```python
from build123d import *

# Parameters (mm, degrees)
F0_W           = 140
F0_H           = 30
F1_DEPTH       = 8
F2_R           = 8.25
F3_DEPTH       = 2
F5_D           = 9
F5_CSINK_D     = 16.5
F5_CSINK_ANGLE = 90
F6_R           = 4
F7_DEPTH       = 55
F8_R           = 2
F10_D          = 6


with BuildPart() as f1:
    # F0 (on Top) → F1 (new body)
    with BuildSketch(Plane.XY):
        Rectangle(F0_W, F0_H)
    extrude(amount=F1_DEPTH)

    # F2 (on face) → F3 (cut)
    with BuildSketch(Plane.XY.offset(8)):
        with Locations((-55, 0)):
            Circle(F2_R)
        Circle(F2_R)
        with Locations((55, 0)):
            Circle(F2_R)
    extrude(amount=-F3_DEPTH, mode=Mode.SUBTRACT)

    # F5 (through all)
    with Locations(Plane.XY.offset(6)):
        with Locations((-55, 0), (0, 0), (55, 0)):
            CounterSinkHole(F5_D / 2, F5_CSINK_D / 2, counter_sink_angle=F5_CSINK_ANGLE)

    # F6 (on Right) → F7 (cut, symmetric)
    with BuildSketch(Plane.YZ):
        with Locations((0, 8)):
            Circle(F6_R)
    extrude(amount=F7_DEPTH, both=True, mode=Mode.SUBTRACT)

    # F8
    f8_edges = [f1.edges().sort_by_distance(p)[0] for p in [
        (-27.5, 4, 8),
        (27.5, 4, 8),
        (27.5, -4, 8),
        (-27.5, -4, 8),
    ]]
    fillet(f8_edges, radius=F8_R)

    # F10 (through all)
    with Locations(Plane.XY.offset(8)):
        with Locations((-40, 0), (40, 0)):
            Hole(F10_D / 2)


solid = f1.part
```
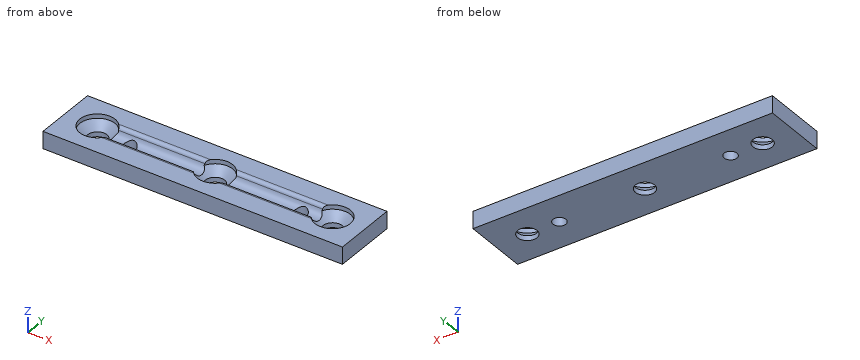
Could you check a few things on this model? Use its own coordinates, in mm. Give positions to 0.01 mm unless a question says otherwise; leave off trailing zeros. Order: outer loops, then holes, each group sorted by start corner. A loop starts at its lowest first (then second) coordinate and runs counter-clockwise, first axis right, second up.
Q1. If I drill on line 1 along X through (y, z) = (0, 0.55); line 2 along Y through (x, z) = (-55, 0.9); line 3 along X through (y, z) = (0, 7.1), over which ranges is the centre line in solid material (lowest first)?
Q2. I'm going to push flat-ended pins straight in: P1, Ø11.5, axis at x = 55, y = 0, coming from the -Z side; P2, Ø7, axis at x = 40, y = 0, coming from the +Z side; P3, Ø5.5, axis at x = -40, y = 0, coming from the +Z side; P4, Ø15, axis at x = 55, y = 0, coming from the +Z side. Where does each tip first touch, or does it pass through?
Q3. Suppose I cut it at B-B, the plane y = 0. Count the separate pieces of the cut face and the enclosed holes in it, and give its area (3 significant figures).
Q4. Suppose I cut it at C-C, the plane x = 40. Write out the boundary of the cut face in (y, z), and give its area (3 significant figures).
Q5. Suppose I cut it at A-A, the plane x = 0. Write out the boundary of the cut face in (y, z), and give its area (3 significant figures).
Solution:
1. line 1: x = -70 to -59.5, -50.5 to -43, -37 to -4.5, 4.5 to 37, 43 to 50.5, 59.5 to 70
1. line 2: y = -15 to -4.5, 4.5 to 15
1. line 3: x = -70 to -63.25, 63.25 to 70
2. P1: stops at z = 0
2. P2: stops at z = 6.06
2. P3: passes through
2. P4: stops at z = 5.25
3. separate pieces: 6
3. enclosed holes: 0
3. area: 453 mm2
4. outline: (-15, 0) - (-3, 0) - (-3, 5.35) arc R4 cw to (-3.77, 6.67) arc R2 ccw to (-5.66, 8) - (-15, 8) - close; (3, 0) - (15, 0) - (15, 8) - (5.66, 8) arc R2 ccw to (3.77, 6.67) arc R4 cw to (3, 5.35) - close
4. area: 187 mm2
5. outline: (-15, 0) - (-4.5, 0) - (-4.5, 2.25) - (-8.25, 6) - (-8.25, 8) - (-15, 8) - close; (4.5, 0) - (15, 0) - (15, 8) - (8.25, 8) - (8.25, 6) - (4.5, 2.25) - close
5. area: 139 mm2
